Verification items for the finished model (mm, model axes). A direction names the side the tool comes from. Round coordinates to 2 decimals unless told otherwise and drop trailing zeros. Loops run counter-clockwise (first coordinate to the right, second up) from the corner with the lowest first, then second, coordinate; pieces in that order, holes last. Notation, with made-up numbers: (-12, -35.5) - (37, -35.5) arc R29 cw to (37, -1.5) - close; hole circle Ø9 at (86.25, -31.75). An arc over 180 degrees is marked (long way). Use a Markdown table: item, result. Add a question column.
```python
from build123d import *

# Parameters (mm, degrees)
CROQUIS1_W              = 700
CROQUIS1_H              = 300
SALIENTE_EXTRUIR1_DEPTH = 200
CROQUIS2_W              = 680
CROQUIS2_H              = 280
CORTAR_EXTRUIR1_DEPTH   = 190
CROQUIS3_R              = 5
CORTAR_EXTRUIR2_DEPTH   = 700


with BuildPart() as part:
    # Croquis1 → Saliente-Extruir1 (new body)
    with BuildSketch(Plane(origin=(0, 0, 0), x_dir=(1, 0, 0), z_dir=(0, 1, 0))):
        Rectangle(CROQUIS1_W, CROQUIS1_H)
    extrude(amount=SALIENTE_EXTRUIR1_DEPTH)

    # Croquis2 → Cortar-Extruir1 (cut)
    with BuildSketch(Plane(origin=(0, 200, 0), x_dir=(1, 0, 0), z_dir=(0, 1, 0))):
        Rectangle(CROQUIS2_W, CROQUIS2_H)
    extrude(amount=-CORTAR_EXTRUIR1_DEPTH, mode=Mode.SUBTRACT)

    # Croquis3 → Cortar-Extruir2 (cut)
    with BuildSketch(Plane(origin=(350, 0, 0), x_dir=(0, 0, -1), z_dir=(1, 0, 0))):
        with Locations((-125, 185)):
            Circle(CROQUIS3_R)
    extrude(amount=-CORTAR_EXTRUIR2_DEPTH, mode=Mode.SUBTRACT)


solid = part.part
```
Q1. Go/stop test with a flat-tipped pin: pin 1 Ø4 at (x, z) = (15.5, -34) entering from +Y. Record where the tip stops, or that it passes through.
Q2. Set-up check for faces 4 (the face through (-5, 99, 150)), 5 (the face through (-5, 10, -2)): record each of +Z, -Z, +X, -X, +Y, -Y from which the full face is reachable in a straight line by a thin tool's end or side.
Q3. Section check B-B on x = -44. Record the cut outline in (y, z), plus the area to 3 significant figures.
Q4. Release check for a two-part mould opening along X. For faces 1 (the face through (-5, 0, -2)), 2 (the face through (-350, 99, 2)), 3 (the face through (-5, 106, 140)) record: +X half, -X half, draft (parallel to the pull), parting line (faces both ways), or undercut.
Q5. Section check A-A on y = 152. Record the cut outline in (x, z).
Q6. Section check C-C on z = -105. Record the cut outline in (x, y).
Q7. Thickness scan on line 1 along X through (y, z) = (102.5, -8.5); line 2 along Z through (x, y) = (-71.5, 101); line 3 along Y through (x, z) = (343.5, 125). Record the ranges inside material, lowest first.
Determined:
| question | item | result |
|---|---|---|
| 1 | pin 1 | stops at y = 10 |
| 2 | face 4 | +Z, +X, -X, +Y, -Y |
| 2 | face 5 | +Y |
| 3 | outline | (0, -150) - (200, -150) - (200, -140) - (10, -140) - (10, 140) - (200, 140) - (200, 150) - (0, 150) - close |
| 3 | area | 6,800 mm² |
| 4 | face 1 | draft |
| 4 | face 2 | -X half |
| 4 | face 3 | undercut |
| 5 | outline | (-350, -150) - (350, -150) - (350, 150) - (-350, 150) - close; hole (-340, -140) - (340, -140) - (340, 140) - (-340, 140) - close |
| 6 | outline | (-350, 0) - (350, 0) - (350, 200) - (340, 200) - (340, 10) - (-340, 10) - (-340, 200) - (-350, 200) - close |
| 7 | line 1 | x = -350 to -340, 340 to 350 |
| 7 | line 2 | z = -150 to -140, 140 to 150 |
| 7 | line 3 | y = 0 to 180, 190 to 200 |
